from build123d import *

# Parameters (mm, degrees)
SKETCH_1_W                  = 80
SKETCH_1_H                  = 345
EXTRUDE_1_DEPTH             = 16
HOLE_WIZARD_16_0_16_1_D     = 16
HOLE_WIZARD_16_0_16_1_DEPTH = 38
HOLE_WIZARD_16_0_16_1_TIP   = 4.806884952
CHAMFER_1_SIZE              = 10
HOLE_WIZARD_16_0_16_2_D     = 34


with BuildPart() as part:
    # 草图1 → 凸台-拉伸1 (new body)
    with BuildSketch(Plane.XY):
        with Locations((40, 172.5)):
            Rectangle(SKETCH_1_W, SKETCH_1_H)
    extrude(amount=EXTRUDE_1_DEPTH)

    # Ø16.0 (16) 直径孔1
    with Locations(Plane.XY.offset(16)):
        with Locations((40, 315), (40, 30)):
            Hole(HOLE_WIZARD_16_0_16_1_D / 2, depth=HOLE_WIZARD_16_0_16_1_DEPTH)
            with Locations((0, 0, -(HOLE_WIZARD_16_0_16_1_DEPTH + HOLE_WIZARD_16_0_16_1_TIP / 2))):  # 118° drill point
                Cone(0, HOLE_WIZARD_16_0_16_1_D / 2, HOLE_WIZARD_16_0_16_1_TIP, mode=Mode.SUBTRACT)

    # 倒角1
    chamfer_1_edges = [part.edges().sort_by_distance(p)[0] for p in [
        (0, 345, 8),
        (80, 345, 8),
        (80, 0, 8),
        (0, 0, 8),
    ]]
    chamfer(chamfer_1_edges, length=CHAMFER_1_SIZE)

    # Ø16.0 (16) 直径孔2 (through all)
    with Locations(Plane.XY.offset(16)):
        with Locations((40, 172.5)):
            Hole(HOLE_WIZARD_16_0_16_2_D / 2)


solid = part.part
Could you check a few things on this model? Use its own coordinates, in mm. Round coordinates to 2 decimals unless told otherwise and drop trailing zeros. Write each loop counter-clockwise with the first axis right and the second up, starting at its lowest first coordinate (ties: lowest second). Pieces come first, ordered by that corner, then holes. Notation, with made-up numbers: (84, 2.25) - (130, 2.25) arc R20 ccw to (130, 7.25) - close; hole circle Ø2 at (13, 51.25). An arc over 180 degrees is marked (long way). Put each result on its own line as item: value. Start each with the question number.
(1) I want a section at D-D, the plane x = 53. Please give me the cut outline in (y, z), plus the area to 3 significant figures.
(2) Thinking about a two-plate mould opening in Y: for faces 1 (the flat face through (40, 0, 8)), 2 (the cylindrical face through (41.041, 322.932, 7.888)), 3 (the flat face through (57, 175, 16)), 4 (the cylindrical face through (41.041, 37.932, 7.888)), which applies, released by +Y, released by -Y, zero draft, split by the parting line, or undercut?
(3) I want a section at B-B, the plane z = 8.75. Please give me the cut outline in (x, y), plus the area to 3 significant figures.
(4) I need wall thicknesses on probe 1 along Y at (x, z) = (40, 10.75); probe 2 along Y at (x, z) = (29.5, 1.25); probe 3 along Y at (x, z) = (45, 4.25) (3 decimals). Which ranges of each line are inside material? Lowest first, please.
(5) I want a section at A-A, the plane y = 172.5. Please give me the cut outline in (x, z), plus the area to 3 significant figures.
(6) I want a section at C-C, the plane x = 40. Please give me the cut outline in (y, z), plus the area to 3 significant figures.
Here are the results:
1. outline: (0, 0) - (161.55, 0) - (161.55, 16) - (0, 16) - close; (183.45, 0) - (345, 0) - (345, 16) - (183.45, 16) - close
1. area: 5,170 mm^2
2. face 1: released by -Y
2. face 2: undercut
2. face 3: zero draft
2. face 4: undercut
3. outline: (0, 10) - (10, 0) - (70, 0) - (80, 10) - (80, 335) - (70, 345) - (10, 345) - (0, 335) - close; hole circle Ø34 at (40, 172.5); hole circle Ø16 at (40, 30); hole circle Ø16 at (40, 315)
3. area: 26,100 mm^2
4. probe 1: y = 0 to 22, 38 to 155.5, 189.5 to 307, 323 to 345
4. probe 2: y = 0 to 159.13, 185.87 to 345
4. probe 3: y = 0 to 23.755, 36.245 to 156.252, 188.748 to 308.755, 321.245 to 345
5. outline: (0, 0) - (23, 0) - (23, 16) - (0, 16) - close; (57, 0) - (80, 0) - (80, 16) - (57, 16) - close
5. area: 736 mm^2
6. outline: (0, 0) - (22, 0) - (22, 16) - (0, 16) - close; (38, 0) - (155.5, 0) - (155.5, 16) - (38, 16) - close; (189.5, 0) - (307, 0) - (307, 16) - (189.5, 16) - close; (323, 0) - (345, 0) - (345, 16) - (323, 16) - close
6. area: 4,460 mm^2
